Design review of the part built by this model. Coordinates are the model's own, in mm. A direction names the side the tool comes from. Coordinates: 2 decimals unless noted, no trailing zeros. Write each loop counter-clockwise with the first axis right and the second up, starting at its lowest first coordinate (ties: lowest second). Pieces come first, ordered by that corner, then holes. Notation, with made-up numbers: M 44.5,6 L 95.5,6 A34 cw 95.5,43 Z; hole C 13,58 d6. An arc over 180 degrees is marked long. Write item = value, one per line.
Autodesk Inventor part; units mm, degrees
ref_plane "YZ Plane" through (0, 0, 0) normal (1, 0, 0) x (0, 1, 0)
ref_plane "XZ Plane" through (0, 0, 0) normal (0, 1, 0) x (-1, 0, 0)
ref_plane "XY Plane" through (0, 0, 0) normal (0, 0, 1) x (1, 0, 0)
sketch "Sketch2" plane through (0, 0, 0) normal (0, 1, 0) x (-1, 0, 0)
  line L0 (0, 0) -> (-15.380673, 0) construction
  line L1 (0, 12) -> (0, -86.646063) construction
  circle A0 centre (0, 0) radius 2
  circle A1 centre (-12, 0) radius 10
  circle A2 centre (-23.313708, -11.313708) radius 6
  circle A3 centre (-16, -32.062435) radius 16
  line L2 (-16, -48.062435) -> (0, -48.062435)
  line L3 (-12, 10) -> (0, 10)
  line L4 (-12, 0) -> (-23.313708, -11.313708)
  arc A4 (-19.562803, 6.542477) -> (-31.877188, -34.041046) centre (19.892258, -27.589553) ccw
  line L5 (0, 0) -> (15.380673, 0) construction
  circle A5 centre (0, 0) radius 2
  circle A6 centre (12, 0) radius 10
  circle A7 centre (23.313708, -11.313708) radius 6
  circle A8 centre (16, -32.062435) radius 16
  line L6 (16, -48.062435) -> (0, -48.062435)
  line L7 (12, 10) -> (0, 10)
  line L8 (12, 0) -> (23.313708, -11.313708)
  arc A9 (31.877188, -34.041046) -> (19.562803, 6.542477) centre (-19.892258, -27.589553) ccw
  arc A10 (10.751933, -47.177256) -> (0, -45.834116) centre (2.223823, -71.738838) ccw
  arc A11 (0, 6.931712) -> (7.2, 8.772685) centre (0, 21.931712) ccw
  arc A12 (0, -45.834116) -> (-10.751933, -47.177256) centre (-2.223823, -71.738838) ccw
  arc A13 (-7.2, 8.772685) -> (0, 6.931712) centre (0, 21.931712) ccw
  line L9 (-23.313708, -11.313708) -> (-58.366086, -46.366086)
  line L10 (-12, 0) -> (-38.351414, 26.351414)
  line L11 (10.154637, -70.237898) -> (-38.67512, -21.408141)
  circle A14 centre (-36.041631, -24.041631) radius 16
  circle A15 centre (-12.425271, -47.65799) radius 16
  circle A16 centre (3.979174, -64.062435) radius 16
  line L12 (0, 10) -> (0, -48.062435)
  point P0 (3.569483, -48.067681)
  point P1 (-12.01558, -63.652744)
  point P2 (-7.2, 8.772685)
  point P3 (-29.089266, -9.631057)
  point P4 (-30.409272, -39.017496)
  point P5 (-10.751933, -47.177256)
  point P6 (-21.637972, -17.07495)
  point P7 (-21.319061, -16.972452)
  point P8 (-21.632358, -17.08657)
  point P9 (-29.07495, -9.637972)
  point P10 (-32.277182, -27.80608)
  point P11 (-31.595554, -28.487707)
  point P12 (0, -45.834116)
  point P13 (-28.928532, -9.198584)
  dimension "d0" = 4
  dimension "d1" = 20
  dimension "d2" = 12
  dimension "d3" = 32
  dimension "d4" = 135
  dimension "d6" = 26
  dimension "d7" = 15
  dimension "d8" = 90
  dimension "d12" = 34
  dimension "d13" = 32
  dimension "d14" = 32
  dimension "d15" = 32
sketch "Sketch9" plane through (0, 0, 0) normal (0, 1, 0) x (-1, 0, 0)
  point P0 (0, 0)
sketch "Sketch2 outline for Extrusion5" plane through (0, 0, 0) normal (0, 1, 0) x (-1, 0, 0)
  arc A0 (3.569483, -48.067681) -> (-12.01558, -63.652744) centre (3.979174, -64.062435) ccw
  arc A1 (-12.01558, -63.652744) -> (3.569483, -48.067681) centre (-12.425271, -47.65799) ccw
extrude "Extrusion5" add sketch "Sketch2 outline for Extrusion5" along normal mid plane 10
fillet "Fillet1" radius 3 4 edges at (7.3345, 5, -52.7487) (1.1116, 5, -58.9717) (7.3345, -5, -52.7487) (1.1116, -5, -58.9717)
sketch "Sketch11" plane through (0, 0, 0) normal (0, 1, 0) x (-1, 0, 0)
  line L0 (0, -51.926604) -> (-2.4, -51.926604)
  line L1 (-2.4, -51.926604) -> (-2.4, -38.067681)
  line L2 (-2.4, -38.067681) -> (0, -38.067681)
  line L3 (0, -38.067681) -> (0, -51.926604)
  arc A0 (-12.01558, -63.652744) -> (3.569483, -48.067681) centre (-12.425271, -47.65799) ccw construction
  line L4 (3.569483, -48.067681) -> (-7.561691, -48.067681)
  point P0 (0, 0)
  dimension "d48" = 10
  dimension "d49" = 4.8
  dimension "d50" = 0
revolve "Revolution3" add sketch "Sketch11" angle 360 about axis through (0, 0, -38.067681) along (0, 0, -1)
chamfer "Chamfer5" distance 1 angle 45 1 edges at (-2.4, 0, -38.0677)
sketch "Sketch5" plane through (0, 0, 0) normal (0, 1, 0) x (-1, 0, 0)
  line L0 (-23.313708, -11.313708) -> (-58.366086, -46.366086) construction
  circle A0 centre (-36.041631, -24.041631) radius 16
  line L1 (-36.041631, -24.041631) -> (-36.041631, 0)
  line L2 (0, 0) -> (0, -9.637972)
  line L3 (-29.07495, -9.637972) -> (29.07495, -9.637972) construction
  line L4 (-36.041631, -24.041631) -> (-36.041631, -40.041631)
  point P0 (-36.041631, -8.041631)
sketch "Sketch6" plane through (0, 0, 0) normal (0, 1, 0) x (-1, 0, 0)
  line L0 (40.788427, -34.041046) -> (-37.176167, -34.041046)
  line L1 (-37.176167, -34.041046) -> (-37.176167, -50.872651)
  line L2 (-37.176167, -50.872651) -> (40.788427, -50.872651)
  line L3 (40.788427, -50.872651) -> (40.788427, -34.041046)
  point P0 (0, 0)
  dimension "d34" = 45
  dimension "d35" = 2
sketch "Sketch3" plane through (0, 0, 0) normal (0, -1, 0) x (1, 0, 0)
  line L0 (-51.381118, -10) -> (56.260395, -10)
  line L1 (56.260395, -10) -> (56.260395, -25)
  line L2 (56.260395, -25) -> (-51.381118, -25)
  line L3 (-51.381118, -25) -> (-51.381118, -10)
  point P0 (0, 0)
  dimension "d22" = 15
  dimension "d23" = 10
properties part number "Apple_logo_red"
Q1. For P1, Ø4, axis at y = -3.5, z = -54, coming from the +X side; P2, Ø5, axis at y = 3.5, z = -52, coming from the -X side; P3, Ø2, axis at y = -1.5, z = -49.5, coming from the -X side, all flat-tipped, find the tip position at first contact; note any pin that passes through.
Check result:
P1 = 9.65
P2 = -3.42
P3 = -3.55
Q2. Consider section A-A, the plane y = 0. State the section outline as (x, z) points.
Check result:
outline = M -3.57,-48.07 A16 ccw 12.02,-63.65 A16 ccw 2.4,-49.39 L 2.4,-39.07 L 1.4,-38.07 L -1.4,-38.07 L -2.4,-39.07 L -2.4,-48.14 A16 ccw Z
Q3. The part is to be moulded in two halves that separate along X. For faces 1 (the flat face through (4, -5, -56)), 2 (the cylindrical face through (9.04, -0.03, -54.76)), 3 (the cylindrical face through (-2.678, -0.028, -48.115)), 4 (the cylindrical face through (0.99, -0.03, -58.85)), say which applies: +X half, -X half, draft (parallel to the pull), parting line (faces both ways), or undercut.
Check result:
face_1 = draft
face_2 = +X half
face_3 = undercut
face_4 = -X half
Q4. Consider section B-B, the plane z = -43. State the section outline as (x, y) points, and give its area (3 significant figures).
Check result:
outline = C 0,0 d4.8
area = 18.1 mm²
Q5. Machinability: for faces 5 (the flat face through (4, 5, -56)), 6 (the cylindrical face through (2.29, 0.72, -44.16)), which of the approach directions +Z, -Z, +X, -X, +Y, -Y give a long, thin tool a straight path to every point of the face, cutting with its end or side? Answer none if there is none.
Check result:
face_5 = +Z, -Z, +X, -X, +Y
face_6 = +Z
Q6. Wall thickness on line 1 (X direction, y = 3, z = -58); line 2 (X direction, y = -4.5, z = -53.75); line 3 (Z direction, x = 5.5, y = 0.5): over which ranges is each line inside the solid? List them lowest first.
Check result:
line_1 = 0.44 to 10.64
line_2 = -0.91 to 6.44
line_3 = -62.08 to -51.17
Q7. Consider section C-C, the plane y = 4.25. State the section outline as (x, z) points.
Check result:
outline = M -2.48,-49.15 A14.98 ccw 10.93,-62.57 A14.98 ccw Z
